```python
from build123d import *

# Parameters (mm, degrees)
F1_DEPTH      = 6.7056
F2_SIZE2      = 0.7366
F2_SIZE       = 1.27
F4_DEPTH      = 25
F4_DEPTH_BACK = 25


with BuildPart() as f1:
    # F0 (on Front) → F1 (new body)
    with BuildSketch(Plane.XZ):
        Polygon((2.0828, 0), (0, 0), (-2.0828, 0), (-3.3528, -0.7366), (0, -4.6228), (3.3528, -0.7366), align=None)
    extrude(amount=F1_DEPTH)

    # F2
    f2_edges = [f1.edges().sort_by_distance(p)[0] for p in [
        (0, -6.7056, 0),
        (0, 0, 0),
    ]]
    chamfer(f2_edges, length=F2_SIZE, length2=F2_SIZE2)

    # F3 (on Right) → F4 (cut, two sides)
    with BuildSketch(Plane.YZ) as f4_sk:
        Polygon((-3.3528, -4.6228), (-6.7056, -0.7366), (-7.370114, -5.010986), (0.519709, -5.010986), (0, -0.7366), align=None)
    extrude(amount=F4_DEPTH, mode=Mode.SUBTRACT)
    extrude(f4_sk.sketch, amount=-F4_DEPTH_BACK, mode=Mode.SUBTRACT)


solid = f1.part
```
Read the model definition and answer for the solid it produces. Units are mm, in the model's axes. Coordinates: 2 decimals unless noted, no trailing zeros. Order: outer loops, then holes, each group sorted by start corner. A loop starts at its lowest first (then second) coordinate and runs counter-clockwise, first axis right, second up. Notation, with made-up numbers: (-4.75, 44) - (-0.75, 44) arc R23 cw to (-0.75, 54) - close; hole circle Ø8 at (-9.5, 44). An arc over 180 degrees is marked (long way). Answer as a JSON object with one key per item and string values. Group by question number.
Item 1: Consider probe 1 along X at (y, z) = (-1.5, -0.4); probe 2 along Y at (x, z) = (-2.75, -1.15); probe 3 along Z at (x, y) = (1, -2.25). Determine where each line is inside the solid, lowest interval first. Write a range as from..to.
Item 2: Flat-ended cylindrical pins translate along their axes: P1, Ø1, axis at x = -1.5, z = -1.5, coming from the -Y side; P2, Ø2, axis at x = -1, z = -4, coming from the +Y side; P3, Ø2, axis at y = -4, z = -2.5, coming from the -X side; P4, Ø2, axis at x = -2, z = -4, coming from the +Y side. Find the tip coordinate at first contact, or state that the pin passes through.
Item 3: Section D-D (z = -3.8) is taken. Give the vertices of the cut face in (x, y).
Item 4: Section C-C (z = -2.25) is taken. Give the vertices of the cut face in (x, y).
Item 5: Section B-B (y = -5.75) is taken. Give the vertices of the cut face in (x, z), plus the area to 3 significant figures.
Item 6: Section A-A (x = -0.5) is taken. Give the vertices of the cut face in (y, z), plus the area to 3 significant figures.
Results are:
{
 "1": {"probe 1": "x = -2.77..2.77", "probe 2": "y = -6.35..-0.36", "probe 3": "z = -3.34..0"},
 "2": {"P1": "stops at y = -6.48", "P2": "stops at y = -1.95", "P3": "stops at x = -2.69", "P4": "passes through"},
 "3": {"outline": "(-0.71, -4.06) - (0.71, -4.06) - (0.71, -2.64) - (-0.71, -2.64) - close"},
 "4": {"outline": "(-2.05, -5.4) - (2.05, -5.4) - (2.05, -1.31) - (-2.05, -1.31) - close"},
 "5": {"outline": "(-3.35, -0.74) - (-2.4, -1.84) - (2.4, -1.84) - (3.35, -0.74) - (2.4, -0.18) - (-2.4, -0.18) - close", "area": "9.56 mm^2"},
 "6": {"outline": "(-6.71, -0.74) - (-3.85, -4.04) - (-2.85, -4.04) - (0, -0.74) - (-1.27, 0) - (-5.44, 0) - close", "area": "16.7 mm^2"}
}
